Here's how the part is built. I have some questions about the finished solid (model axes, mm). Face numbers are marked on the shaded views. Round coordinates to 2 decimals unless told otherwise and drop trailing zeros. Loops run counter-clockwise (first coordinate to the right, second up) from the corner with the lowest first, then second, coordinate; pieces in that order, holes last. Notation, with made-up numbers: M 28.25,-30.75 L 35.25,-30.75 A22 ccw 35.25,-10.75 Z; hole C -10,46 d10. An arc over 180 degrees is marked long. Answer as a JSON object with one key per item and string values.
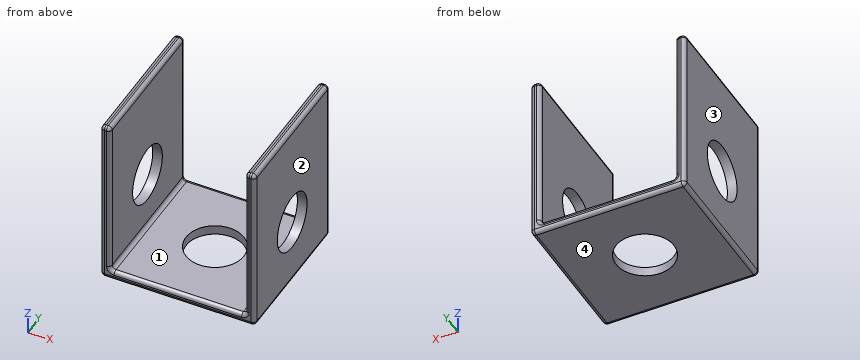
from build123d import *

# Parameters (mm, degrees)
SKETCH1_W           = 80
SKETCH1_H           = 90
BOSS_EXTRUDE1_DEPTH = 75
SKETCH2_W           = 70
SKETCH2_H           = 85
CUT_EXTRUDE2_DEPTH  = 142.862609591
SKETCH3_R           = 15
CUT_EXTRUDE3_DEPTH  = 142.862609591
SKETCH4_R           = 15
CUT_EXTRUDE4_DEPTH  = 139.744369255
FILLET1_R           = 2


with BuildPart() as part:
    # Sketch1 → Boss-Extrude1 (new body)
    with BuildSketch(Plane(origin=(0, 0, 0), x_dir=(1, 0, 0), z_dir=(0, 1, 0))):
        with Locations((40, 45)):
            Rectangle(SKETCH1_W, SKETCH1_H)
    extrude(amount=BOSS_EXTRUDE1_DEPTH)

    # Sketch2 → Cut-Extrude2 (cut, through all)
    with BuildSketch(Plane(origin=(0, 75, 0), x_dir=(1, 0, 0), z_dir=(0, 1, 0))):
        with Locations((40, 42.5)):
            Rectangle(SKETCH2_W, SKETCH2_H)
    extrude(amount=-CUT_EXTRUDE2_DEPTH, mode=Mode.SUBTRACT)

    # Sketch3 → Cut-Extrude3 (cut, through all)
    with BuildSketch(Plane.ZY):
        with Locations((-55, 37.5)):
            Circle(SKETCH3_R)
    extrude(amount=-CUT_EXTRUDE3_DEPTH, mode=Mode.SUBTRACT)

    # Sketch4 → Cut-Extrude4 (cut, through all)
    with BuildSketch(Plane.XY.offset(-85)):
        with Locations((40, 37.5)):
            Circle(SKETCH4_R)
    extrude(amount=-CUT_EXTRUDE4_DEPTH, mode=Mode.SUBTRACT)

    # Fillet1
    fillet1_edges = [part.edges().sort_by_distance(p)[0] for p in [
        (80, 75, -45),
        (77.5, 0, 0),
        (40, 75, -90),
        (77.5, 75, 0),
        (75, 37.5, 0),
        (5, 0, -42.5),
        (5, 37.5, 0),
        (40, 0, -85),
        (5, 37.5, -85),
        (75, 0, -42.5),
        (75, 37.5, -85),
        (75, 75, -42.5),
        (40, 75, -85),
        (5, 75, -42.5),
        (0, 75, -45),
        (40, 0, -90),
        (80, 0, -45),
        (2.5, 0, 0),
        (0, 0, -45),
        (0, 37.5, -90),
        (80, 37.5, -90),
        (80, 37.5, 0),
        (0, 37.5, 0),
        (2.5, 75, 0),
    ]]
    fillet(fillet1_edges, radius=FILLET1_R)


solid = part.part
Item 1: I want a section at D-D, the plane z = -55. Please give me the cut outline in (x, y), then the cut area to 3 significant figures.
Resolved:
{"outline": "M 0,2 A2 ccw 2,0 L 3,0 A2 ccw 5,2 L 5,22.5 L 0,22.5 Z; M 0,52.5 L 5,52.5 L 5,73 A2 ccw 3,75 L 2,75 A2 ccw 0,73 Z; M 75,2 A2 ccw 77,0 L 78,0 A2 ccw 80,2 L 80,22.5 L 75,22.5 Z; M 75,52.5 L 80,52.5 L 80,73 A2 ccw 78,75 L 77,75 A2 ccw 75,73 Z", "area": "443 mm²"}
Item 2: If we mould it in two halves opening along X, with no side actions, what happens to the marked faces 1, 2, 3 and 4? For each: pulls with the +X half, pulls with the -X half, needs draft (parallel to the pull), parting line crosses it, or undercut.
Resolved:
{"face 1": "undercut", "face 2": "pulls with the +X half", "face 3": "pulls with the -X half", "face 4": "needs draft"}
Item 3: I want a section at B-B, the plane y = 37.5. Please give me the cut outline in (x, z), then the cut area to 3 significant figures.
Resolved:
{"outline": "M 0,-88 A2 ccw 2,-90 L 25,-90 L 25,-85 L 7,-85 A2 cw 5,-83 L 5,-70 L 0,-70 Z; M 0,-40 L 5,-40 L 5,-2 A2 ccw 3,0 L 2,0 A2 ccw 0,-2 Z; M 55,-90 L 78,-90 A2 ccw 80,-88 L 80,-70 L 75,-70 L 75,-83 A2 cw 73,-85 L 55,-85 Z; M 75,-40 L 80,-40 L 80,-2 A2 ccw 78,0 L 77,0 A2 ccw 75,-2 Z", "area": "797 mm²"}
Item 4: I'm going to push a flat-ended pin straight in: pin 1 Ø1.5 at (x, y) = (49, 16) entering from +Z. Where does the tip first touch, or does it pass through?
Resolved:
{"pin 1": "z = -85"}
Item 5: Please list where these lines run through material, in increasing order: probe 1 along X at (y, z) = (4.5, -57); probe 2 along Z at (x, y) = (2, 37); probe 3 along Y at (x, z) = (40, -88.25). Write a range as from..to.
Resolved:
{"probe 1": "0..5, 75..80", "probe 2": "-90..-69.99, -40.01..0", "probe 3": "0.02..22.5, 52.5..74.98"}
Item 6: I want a section at C-C, the plane x = 40. Please give me the cut outline in (y, z).
Resolved:
{"outline": "M 0,-88 A2 ccw 2,-90 L 22.5,-90 L 22.5,-85 L 2,-85 A2 ccw 0,-87 Z; M 52.5,-90 L 73,-90 A2 ccw 75,-88 L 75,-87 A2 ccw 73,-85 L 52.5,-85 Z"}
Item 7: I want a section at A-A, the plane z = -74. Please give me the cut outline in (x, y), then the cut area to 3 significant figures.
Resolved:
{"outline": "M 0,2 A2 ccw 2,0 L 3,0 A2 ccw 5,2 L 5,73 A2 ccw 3,75 L 2,75 A2 ccw 0,73 Z; M 75,2 A2 ccw 77,0 L 78,0 A2 ccw 80,2 L 80,73 A2 ccw 78,75 L 77,75 A2 ccw 75,73 Z", "area": "743 mm²"}
